Design review of the part built by this model. Coordinates are the model's own, in mm. Round coordinates to 2 decimals unless told otherwise and drop trailing zeros. Order: outer loops, then holes, each group sorted by start corner. A loop starts at its lowest first (then second) coordinate and runs counter-clockwise, first axis right, second up.
from build123d import *

# Parameters (mm, degrees)
F1_DEPTH = 25
F2_D     = 2


with BuildPart() as f1:
    # F0 (on Top) → F1 (new body)
    with BuildSketch(Plane.XY):
        with BuildLine():
            ThreePointArc((0, 11.6000010935), (-2, 9.6000010935), (0, 7.6000010935))
            Line((0, 7.6000010935), (17.5, 7.6000010935))
            ThreePointArc((17.5, 7.6000010935), (19.5, 9.6000010935), (17.5, 11.6000010935))
            Line((17.5, 11.6000010935), (0, 11.6000010935))
        make_face()
    extrude(amount=F1_DEPTH)

    # F2 (through all)
    with Locations(Plane(origin=(0, 0, 0), x_dir=(1, 0, 0), z_dir=(0, 0, -1))):
        with Locations((0, -9.6000010935), (2.5, -9.6000010935), (5, -9.6000010935), (7.5, -9.6000010935), (10, -9.6000010935), (12.5, -9.6000010935), (15, -9.6000010935), (17.5, -9.6000010935)):
            Hole(F2_D / 2)


solid = f1.part
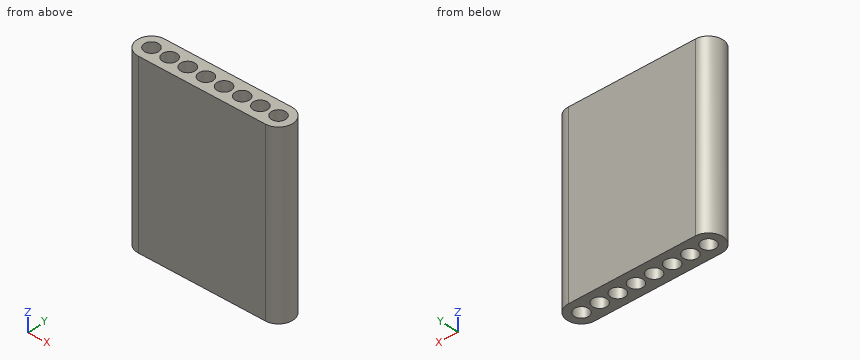
1) Clearance check with flat-ended pins moving along their axes: P1, Ø1.8, axis at x = 15, y = 9.6, coming from the +Z side; P2, Ø1.5, axis at y = 8.5, z = 6, coming from the +X side. State where each tip first meets the part, or that it passes through.
Results:
P1: passes through
P2: stops at x = 19.47
2) Take a section at D-D on y = 11.2. Give the boundary of the cut face in (x, z).
Results:
outline: (-1.2, 0) - (18.7, 0) - (18.7, 25) - (-1.2, 25) - close
3) Take a section at B-B on z = 13.5. State how many separate pieces and enclosed holes the cut face has, plus the area to 3 significant figures.
Results:
separate pieces: 1
enclosed holes: 8
area: 57.4 mm2
4) Take a section at C-C on x = 10.25. Give the boundary of the cut face in (y, z).
Results:
outline: (7.6, 0) - (8.63, 0) - (8.63, 25) - (7.6, 25) - close; (10.57, 0) - (11.6, 0) - (11.6, 25) - (10.57, 25) - close
5) Take a section at A-A on x = 7.5. Give the boundary of the cut face in (y, z).
Results:
outline: (7.6, 0) - (8.6, 0) - (8.6, 25) - (7.6, 25) - close; (10.6, 0) - (11.6, 0) - (11.6, 25) - (10.6, 25) - close
6) To check wall thickness, follow line 1 along Y through (x, z) = (15, 10.5); line 2 along Y through (x, z) = (14.5, 9.75); line 3 along X through (y, z) = (8.15, 1.25). State the ranges of each line that lie inside material, in increasing order.
Results:
line 1: y = 7.6 to 8.6, 10.6 to 11.6
line 2: y = 7.6 to 8.73, 10.47 to 11.6
line 3: x = -1.38 to 18.88
